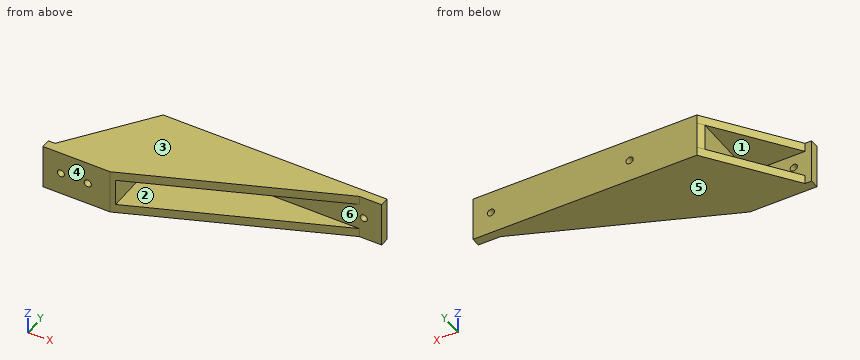
```python
from build123d import *

# Parameters (mm, degrees)
BOSS_EXTRUDE1_DEPTH = 2
SKETCH2_W           = 50
SKETCH2_H           = 10
BOSS_EXTRUDE2_DEPTH = 2
SKETCH3_W           = 15
SKETCH3_H           = 10
BOSS_EXTRUDE3_DEPTH = 2
BOSS_EXTRUDE4_DEPTH = 2
BOSS_EXTRUDE5_DEPTH = 6
SKETCH7_R           = 0.8
CUT_EXTRUDE1_DEPTH  = 20


with BuildPart() as part:
    # Sketch1 → Boss-Extrude1 (new body)
    with BuildSketch(Plane.XY):
        Polygon((0, 0), (-15, 0), (0, 20), (50, 20), align=None)
    extrude(amount=BOSS_EXTRUDE1_DEPTH)

    # Sketch2 → Boss-Extrude2 (add)
    with BuildSketch(Plane(origin=(0, 20, 0), x_dir=(1, 0, 0), z_dir=(0, 1, 0))):
        with Locations((25, 3)):
            Rectangle(SKETCH2_W, SKETCH2_H)
    extrude(amount=-BOSS_EXTRUDE2_DEPTH)

    # Sketch3 → Boss-Extrude3 (add)
    with BuildSketch(Plane.XZ):
        with Locations((-7.5, -3)):
            Rectangle(SKETCH3_W, SKETCH3_H)
    extrude(amount=-BOSS_EXTRUDE3_DEPTH)

    # Sketch4 → Boss-Extrude4 (add)
    with BuildSketch(Plane(origin=(0, 0, -8), x_dir=(-1, 0, 0), z_dir=(0, 0, -1))):
        Polygon((-50, 20), (0, 0), (15, 0), (0, 20), align=None)
    extrude(amount=-BOSS_EXTRUDE4_DEPTH)

    # Sketch6 → Boss-Extrude5 (add)
    with BuildSketch(Plane(origin=(0, 0, 0), x_dir=(-1, 0, 0), z_dir=(0, 0, -1))):
        Polygon((0, 20), (0, 18), (-1, 18), (-1, 0.4), (0, 0), (0, 2), (1, 2), (1, 18.666666667), align=None)
    extrude(amount=BOSS_EXTRUDE5_DEPTH)

    # Sketch7 → Cut-Extrude1 (cut)
    with BuildSketch(Plane(origin=(0, 20, 0), x_dir=(1, 0, 0), z_dir=(0, 1, 0))):
        with Locations(Location((46, 3, 0), (0, 0, 270))):
            Circle(SKETCH7_R)
        with Locations(Location((15, 3, 0), (0, 0, 270))):
            Circle(SKETCH7_R)
        with Locations(Location((-11, 3, 0), (0, 0, 270))):
            Circle(SKETCH7_R)
        with Locations(Location((-5, 3, 0), (0, 0, 270))):
            Circle(SKETCH7_R)
    extrude(amount=-CUT_EXTRUDE1_DEPTH, mode=Mode.SUBTRACT)


solid = part.part
```
Model file for the job. Use its own axes, mm. Face numbers are marked on the shaded views. A direction names the side the tool comes from. Give positions to 0.01 mm unless a question says otherwise; leave off trailing zeros. Loops run counter-clockwise (first coordinate to the right, second up) from the corner with the lowest first, then second, coordinate; pieces in that order, holes last. Notation, with made-up numbers: (7.25, -7) -> (44.25, -7) arc R18 cw to (44.25, 5) -> close; hole circle Ø5 at (-16, 20). An arc over 180 degrees is marked (long way). Write each question's results on one line, items separated by ' | '.
(1) Probe line 1 along X through (y, z) = (0.8, -3); line 2 along Z through (x, y) = (9, 6.5); line 3 along X through (y, z) = (19, -3). List the from-to ranges inside material, lowest first.
Geometry results:
line 1: x = -15 to -11.8, -10.2 to -5.8, -4.2 to 1 | line 2: z = -8 to -6, 0 to 2 | line 3: x = -0.75 to 14.2, 15.8 to 45.2, 46.8 to 50
(2) Pull direction Z, two halves, no side cores. Call the marked faces 4, 5 and 6: released by +Z, released by -Z, zero draft, split by the parting line, or undercut.
Geometry results:
face 4: zero draft | face 5: released by -Z | face 6: undercut
(3) Cut at D-D on x = 36. List the corners of the cut face in (y, z).
Geometry results:
outline: (14.4, -8) -> (20, -8) -> (20, 2) -> (14.4, 2) -> (14.4, 0) -> (18, 0) -> (18, -6) -> (14.4, -6) -> close
(4) Tool access for the marked faces 1, 2 and 3: list every direction of +Z, -Z, +X, -X, +Y, -Y with a clear straight run to the whole face (end or side of a thin tool).
Geometry results:
face 1: -X, +Y | face 2: +X, -Y | face 3: +Z, +X, -X, +Y, -Y
(5) Flat gauge pins, fed straight in: pin 1 Ø1.8 at (y, z) = (8.5, -3) entering from -X; pin 2 Ø5 at (y, z) = (3.5, -6) entering from +X; pin 3 Ø3 at (y, z) = (5.5, -2.5) entering from +X. Where does each tip first touch, or does it go through?
Geometry results:
pin 1: stops at x = -1 | pin 2: stops at x = 15 | pin 3: stops at x = 1
(6) Cut at C-C on y = 10. List the corners of the cut face in (x, z), and give its area (3 significant figures).
Geometry results:
outline: (-7.5, -8) -> (25, -8) -> (25, -6) -> (1, -6) -> (1, 0) -> (25, 0) -> (25, 2) -> (-7.5, 2) -> (-7.5, 0) -> (-1, 0) -> (-1, -6) -> (-7.5, -6) -> close | area: 142 mm²
(7) Cut at A-A on x = 15. List the corners of the cut face in (y, z), and give its area (3 significant figures).
Geometry results:
outline: (6, -8) -> (20, -8) -> (20, -3.8) -> (18, -3.8) -> (18, -6) -> (6, -6) -> close; (6, 0) -> (18, 0) -> (18, -2.2) -> (20, -2.2) -> (20, 2) -> (6, 2) -> close | area: 64.8 mm²
(8) Cut at B-B on z = -3. List the corners of the cut face in (x, y), and give its area (3 significant figures).
Geometry results:
outline: (-15, 0) -> (-11.8, 0) -> (-11.8, 2) -> (-15, 2) -> close; (-10.2, 0) -> (-5.8, 0) -> (-5.8, 2) -> (-10.2, 2) -> close; (-4.2, 0) -> (0, 0) -> (1, 0.4) -> (1, 18) -> (14.2, 18) -> (14.2, 20) -> (0, 20) -> (-1, 18.67) -> (-1, 2) -> (-4.2, 2) -> close; (15.8, 18) -> (45.2, 18) -> (45.2, 20) -> (15.8, 20) -> close; (46.8, 18) -> (50, 18) -> (50, 20) -> (46.8, 20) -> close | area: 152 mm²
